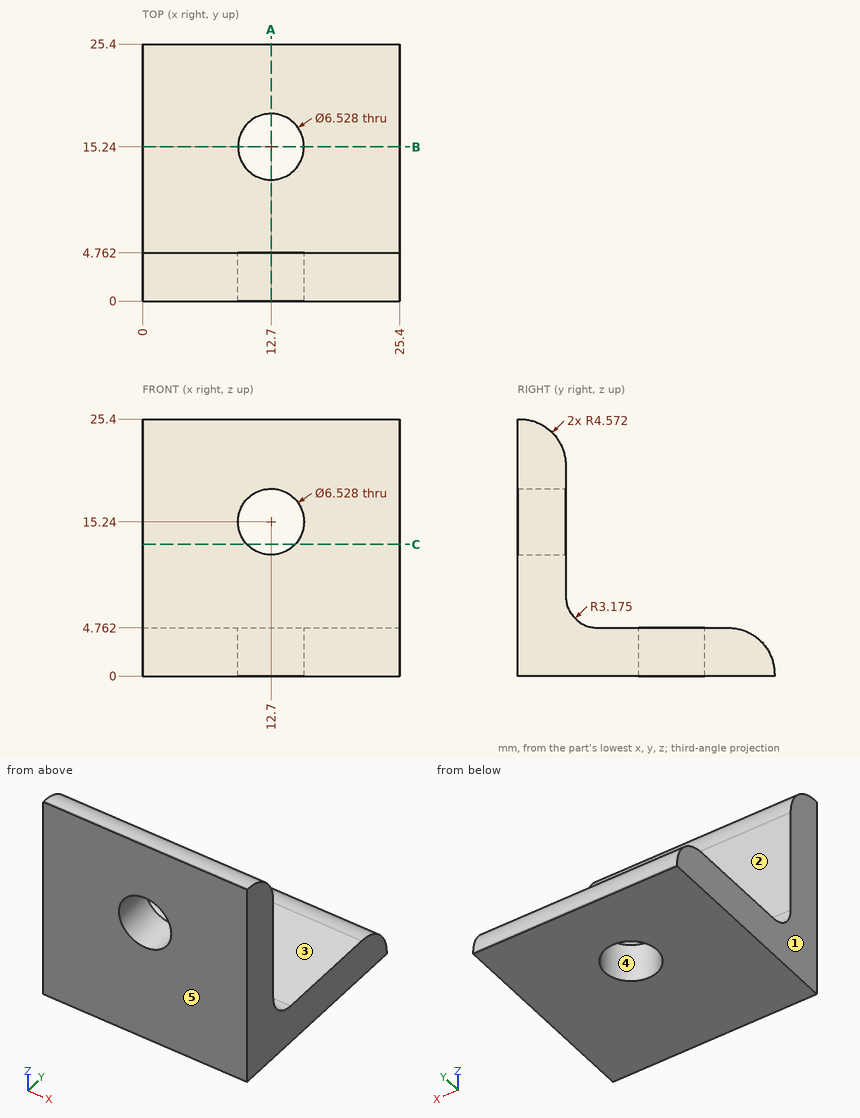
The figure shows three views and two pictorial views of one solid part (mm, origin at its lowest corner). Answer the questions. A direction names the side the tool comes from. Coordinates: 2 decimals unless noted, no trailing zeros. Write each loop counter-clockwise with the first axis right and the second up, starting at its lowest first coordinate (ties: lowest second). Pieces come first, ordered by that corner, then holes. Notation, with made-up numbers: M 42.5,84.5 L 60.5,84.5 A18 cw 60.5,95.5 Z; hole C 68,11 d7. An arc over 180 degrees is marked long. Answer as CSV lines item,"result". Start each with the question number.
Item 1: A tool of negligible diameter and unlimited length cuts with its end or side. For the marked faces 1 and 2, from which of +Z, -Z, +X, -X, +Y, -Y can it reach the whole face along a straight path? Write none if from no direction.
Item 2: Section C-C on z = 13 is taken. Write down the section's boundary in (x, y).
Item 3: Section B-B on y = 15.24 is taken. Write down the section's boundary in (x, z).
Item 4: Section A-A on x = 12.7 is taken. Give the number of separate pieces and of enclosed holes in the cut face, and give its area (3 significant figures).
Item 5: Determine the mould class of the marked faces 3, 4 and 5 for opening direction Y: released by +Y, released by -Y, zero draft, split by the parting line, or undercut.
Item 6: Consider L1, parallel to X at y = 3.5, z = 15.24; L2, parallel to Z at x = 3, y = 17.75. Determine where each line is inside the solid, lowest interval first.
Item 7: Flat-ended cylindrical pins translate along their axes: P1, Ø6, axis at x = 8.5, y = 6, coming from the +Z side (1 decimal); P2, Ø8, axis at x = 22.5, y = 15.5, coming from the -Z side; P3, Ø12, axis at x = 11.5, z = 16.5, coming from the +Y side; P4, Ø8, axis at x = 17.5, y = 21, coming from the +Z side. Find the tip coordinate at first contact, or state that the pin passes through.
Checks:
1,face 1,"+Z, -Z, -X, +Y, -Y"
1,face 2,"+Z, +X, -X, +Y"
2,outline,"M 0,0 L 10.33,0 L 10.33,4.76 L 0,4.76 Z; M 15.07,0 L 25.4,0 L 25.4,4.76 L 15.07,4.76 Z"
3,outline,"M 0,0 L 9.44,0 L 9.44,4.76 L 0,4.76 Z; M 15.96,0 L 25.4,0 L 25.4,4.76 L 15.96,4.76 Z"
4,separate pieces,"3"
4,enclosed holes,"0"
4,area,"150 mm²"
5,face 3,"zero draft"
5,face 4,"undercut"
5,face 5,"released by -Y"
6,L1,"x = 0 to 9.44, 15.96 to 25.4"
6,L2,"z = 0 to 4.76"
7,P1,"stops at z = 24.4"
7,P2,"stops at z = 0"
7,P3,"stops at y = 4.76"
7,P4,"stops at z = 4.76"
